For this review, take the finished solid that the model builds, in its own axes (mm). A direction names the side the tool comes from. Round coordinates to 2 decimals unless told otherwise and drop trailing zeros. Write each loop counter-clockwise with the first axis right and the second up, starting at its lowest first coordinate (ties: lowest second). Pieces come first, ordered by that corner, then holes. Notation, with made-up numbers: (-21.5, 60.5) -> (33.5, 60.5) arc R13 ccw to (33.5, 66.5) -> close; hole circle Ø9 at (-10, -18.5). An arc over 180 degrees is marked (long way). Answer in a Markdown table with one row per item.
Autodesk Inventor part; units mm, degrees
ref_plane "YZ Plane" through (0, 0, 0) normal (1, 0, 0) x (0, 1, 0)
ref_plane "XZ Plane" through (0, 0, 0) normal (0, 1, 0) x (-1, 0, 0)
ref_plane "XY Plane" through (0, 0, 0) normal (0, 0, 1) x (1, 0, 0)
sketch "Boceto1" plane through (0, 0, 0) normal (0, 0, 1) x (1, 0, 0)
  line L0 (0, 0) -> (43, 0)
  line L1 (43, 0) -> (43, 21)
  line L2 (43, 21) -> (40, 21)
  line L3 (40, 21) -> (40, 3)
  line L4 (40, 3) -> (3, 3)
  line L5 (3, 3) -> (3, 21)
  line L6 (3, 21) -> (0, 21)
  line L7 (0, 21) -> (0, 0)
extrude "Extrusión1" add sketch "Boceto1" against normal blind 35
fillet "Empalme1" radius 5 4 edges at (1.5, 21, 0) (1.5, 21, -35) (41.5, 21, 0) (41.5, 21, -35)
sketch "Boceto2" plane through (43, 0, 0) normal (1, 0, 0) x (0, 0, -1)
  arc A0 (5, 21) -> (0, 16) centre (5, 16) ccw
  circle A1 centre (5, 12) radius 2.5
  circle A2 centre (30, 12) radius 2.5
  point P0 (0, 0)
hole "Agujero1" at (43, 12, -5) at (43, 12, -30) direction (-1, 0, 0) diameter 5 end through all
sketch "Boceto3" plane through (3, 3, 0) normal (0, 1, 0) x (1, 0, 0)
  line L0 (7.25, 23.5) -> (29.75, 23.5)
  line L1 (29.75, 23.5) -> (29.75, 11.5)
  line L2 (29.75, 11.5) -> (7.25, 11.5)
  line L3 (7.25, 11.5) -> (7.25, 23.5)
  point P0 (-3, 0)
  point P1 (0, 35)
extrude "Extrusión2" cut sketch "Boceto3" against normal blind 35
sketch "Boceto4" plane through (3, 3, 0) normal (0, 1, 0) x (1, 0, 0)
  circle A0 centre (32.25, 17.5) radius 1.25
  circle A1 centre (4.75, 17.5) radius 1.25
  point P0 (-3, 0)
hole "Agujero2" at (7.75, 3, -17.5) at (35.25, 3, -17.5) direction (0, -1, 0) diameter 2.5 end through all
properties part number "8"
1) Consider section C-C on y = 12. State the section outline as (x, z) points, then the cut area to 3 significant figures.
Solved:
| item | result |
|---|---|
| outline | (0, -35) -> (3, -35) -> (3, -32.5) -> (0, -32.5) -> close; (0, -27.5) -> (3, -27.5) -> (3, -7.5) -> (0, -7.5) -> close; (0, -2.5) -> (3, -2.5) -> (3, 0) -> (0, 0) -> close; (40, -35) -> (43, -35) -> (43, -32.5) -> (40, -32.5) -> close; (40, -27.5) -> (43, -27.5) -> (43, -7.5) -> (40, -7.5) -> close; (40, -2.5) -> (43, -2.5) -> (43, 0) -> (40, 0) -> close |
| area | 150 mm² |
2) Consider section A-A on x = 34.5. State the section outline as (y, z) points.
Solved:
| item | result |
|---|---|
| outline | (0, -35) -> (3, -35) -> (3, -18.5) -> (0, -18.5) -> close; (0, -16.5) -> (3, -16.5) -> (3, 0) -> (0, 0) -> close |
3) Consider section B-B on y = 6.75. State the section outline as (x, z) points.
Solved:
| item | result |
|---|---|
| outline | (0, -35) -> (3, -35) -> (3, 0) -> (0, 0) -> close; (40, -35) -> (43, -35) -> (43, 0) -> (40, 0) -> close |
4) For line 1 (Z direction, x = 41.05, y = 12); line 2 (X direction, y = 2.1, z = -17.5); line 3 (X direction, y = 19.75, z = -21), list the stretches that pass through material, from the lowest coordinate up. Write a range as [from, to].
Solved:
| item | result |
|---|---|
| line 1 | [-35, -32.5], [-27.5, -7.5], [-2.5, 0] |
| line 2 | [0, 6.5], [9, 10.25], [32.75, 34], [36.5, 43] |
| line 3 | [0, 3], [40, 43] |
5) Clearance check with flat-ended pins moving along their axes: pin 1 Ø10.5 at (x, z) = (13.5, -21.5) entering from +Y; pin 2 Ø3 at (y, z) = (2.5, -30.5) entering from -X; pin 3 Ø3 at (y, z) = (12, -5) entering from +X. State where each tip first meets the part, or that it passes through.
Solved:
| item | result |
|---|---|
| pin 1 | y = 3 |
| pin 2 | x = 0 |
| pin 3 | through |
6) Mouldability with a two-part tool opening along Z and no side actions: class faces 1 (the cylindrical face through (1, 19, -1)), 2 (the flat face through (21.2, 2.8, -35)), 3 (the flat face through (43, 10, -17)), 4 (the flat face through (21, 2, -23.5)) as pulls with the +Z half, pulls with the -Z half, needs draft (parallel to the pull), parting line crosses it, or undercut.
Solved:
| item | result |
|---|---|
| face 1 | pulls with the +Z half |
| face 2 | pulls with the -Z half |
| face 3 | needs draft |
| face 4 | undercut |
7) For faces 5 (the flat face through (22, 3, -9)), 6 (the flat face through (32.75, 2, -18)), 7 (the cylindrical face through (41.48, 14.44, -29.46)), list the 3-axis set-ups (+Z, -Z, +X, -X, +Y, -Y) from which the entire face can be reached by the end or side of a thin tool; tool diameter is ignored.
Solved:
| item | result |
|---|---|
| face 5 | +Z, -Z, +Y |
| face 6 | +Y, -Y |
| face 7 | +X, -X |
8) Consider section D-D on z = -17.5. State the section outline as (x, y) points.
Solved:
| item | result |
|---|---|
| outline | (0, 0) -> (6.5, 0) -> (6.5, 3) -> (3, 3) -> (3, 21) -> (0, 21) -> close; (9, 0) -> (10.25, 0) -> (10.25, 3) -> (9, 3) -> close; (32.75, 0) -> (34, 0) -> (34, 3) -> (32.75, 3) -> close; (36.5, 0) -> (43, 0) -> (43, 21) -> (40, 21) -> (40, 3) -> (36.5, 3) -> close |
